```python
from build123d import *

# Parameters (mm, degrees)
SKETCH1_R           = 4.75
SKETCH1_R_2         = 1.5
BOSS_EXTRUDE1_DEPTH = 2
CHAMFER1_SIZE       = 1.5


with BuildPart() as part:
    # Sketch1 → Boss-Extrude1 (new body)
    with BuildSketch(Plane(origin=(0, 0, 0), x_dir=(1, 0, 0), z_dir=(0, 1, 0))):
        with BuildLine():
            Line((3.5, 17), (3.5, 9.5))
            ThreePointArc((3.5, 9.5), (5.257359313, 5.257359313), (9.5, 3.5))
            Line((9.5, 3.5), (17, 3.5))
            ThreePointArc((17, 3.5), (20.5, 0), (17, -3.5))
            Line((17, -3.5), (9.5, -3.5))
            ThreePointArc((9.5, -3.5), (5.257359313, -5.257359313), (3.5, -9.5))
            Line((3.5, -9.5), (3.5, -17))
            ThreePointArc((3.5, -17), (0, -20.5), (-3.5, -17))
            Line((-3.5, -17), (-3.5, -9.5))
            ThreePointArc((-3.5, -9.5), (-5.257359313, -5.257359313), (-9.5, -3.5))
            Line((-9.5, -3.5), (-17, -3.5))
            ThreePointArc((-17, -3.5), (-20.5, 0), (-17, 3.5))
            Line((-17, 3.5), (-9.5, 3.5))
            ThreePointArc((-9.5, 3.5), (-5.257359313, 5.257359313), (-3.5, 9.5))
            Line((-3.5, 9.5), (-3.5, 17))
            ThreePointArc((-3.5, 17), (0, 20.5), (3.5, 17))
        make_face()
        Circle(SKETCH1_R, mode=Mode.SUBTRACT)
        with Locations((0, 8)):
            Circle(SKETCH1_R_2, mode=Mode.SUBTRACT)
        with Locations((0, 17)):
            Circle(SKETCH1_R_2, mode=Mode.SUBTRACT)
        with Locations((17, 0)):
            Circle(SKETCH1_R_2, mode=Mode.SUBTRACT)
        with Locations((9.5, 0)):
            Circle(SKETCH1_R_2, mode=Mode.SUBTRACT)
        with Locations((0, -17)):
            Circle(SKETCH1_R_2, mode=Mode.SUBTRACT)
        with Locations((0, -8)):
            Circle(SKETCH1_R_2, mode=Mode.SUBTRACT)
        with Locations((-17, 0)):
            Circle(SKETCH1_R_2, mode=Mode.SUBTRACT)
        with Locations((-9.5, 0)):
            Circle(SKETCH1_R_2, mode=Mode.SUBTRACT)
    extrude(amount=BOSS_EXTRUDE1_DEPTH)

    # Chamfer1
    chamfer1_edges = [part.edges().sort_by_distance(p)[0] for p in [
        (-1.5, 2, -8),
        (8, 2, 0),
        (-1.5, 2, 8),
        (-11, 2, 0),
    ]]
    chamfer(chamfer1_edges, length=CHAMFER1_SIZE)


solid = part.part
```
The listing builds one solid part. Answer for the finished solid, in the listing's coordinates (mm). A direction names the side the tool comes from. Coordinates: 2 decimals unless noted, no trailing zeros. Loops run counter-clockwise (first coordinate to the right, second up) from the corner with the lowest first, then second, coordinate; pieces in that order, holes last. Notation, with made-up numbers: (30.5, 57.25) -> (81.5, 57.25) arc R25 cw to (81.5, 79.25) -> close; hole circle Ø1 at (20, -10.5). An arc over 180 degrees is marked (long way). Use one line per item in the form item = value. Start each with the question number.
Item 1: The part is cut by section B-B on x = -18. Determine the outline of the cut face in (y, z).
Item 2: The part is cut by section C-C on z = -8. Determine the outline of the cut face in (x, y).
Item 3: Flat-ended cylindrical pins translate along their axes: pin 1 Ø2.5 at (x, z) = (0, -17) entering from -Y; pin 2 Ø1 at (x, y) = (15, 1) entering from -Z; pin 3 Ø4 at (x, z) = (-17, 0) entering from +Y; pin 4 Ø0.6 at (y, z) = (1.5, -14) entering from -X. Find the tip coordinate at first contact, or state that the pin passes through.
Item 4: The mould has two halves that part along X. Classify faces 6 (the face through (-20.5, 1, 0.1)), 7 (the face through (0, 1, 6)), 8 (the face through (5, 0, -2)): released by +X, released by -X, zero draft, split by the parting line, or undercut.
Item 5: A tool of negligible diameter and unlimited length cuts with its end or side. For faces 1 (the face through (-11, 0.25, -0.07)), 2 (the face through (-13, 1, -3.5)), 3 (the face through (3.5, 1, -13)), 4 (the face through (3.5, 1, 13)), 5 (the face through (-13, 1, 3.5)), from which of +Z, -Z, +X, -X, +Y, -Y can it reach the whole face along a straight path? Write none if from no direction.
Item 6: The part is cut by section A-A on y = 0.85. Count the separate pieces of the cut face and the enclosed holes in it, then the cut area to 3 significant figures.
Item 7: Consider L1, parallel to Z at x = 0.5, y = 0.85; L2, parallel to Z at x = -17, y = 0.1; L3, parallel to X at y = 0.35, z = -8. Determine where each line is inside the solid, lowest interval first. Write a range as [from, to].
Item 8: The part is cut by section D-D on x = 16.5. Determine the outline of the cut face in (y, z).
Answer key:
q1.outline = (0, -3.35) -> (2, -3.35) -> (2, -1.12) -> (0, -1.12) -> close; (0, 1.12) -> (2, 1.12) -> (2, 3.35) -> (0, 3.35) -> close
q2.outline = (-3.69, 0) -> (-1.5, 0) -> (-1.5, 0.5) -> (-3, 2) -> (-3.69, 2) -> close; (1.5, 0) -> (3.69, 0) -> (3.69, 2) -> (3, 2) -> (1.5, 0.5) -> close
q3.pin_1 = through
q3.pin_2 = -3.5
q3.pin_3 = 2
q3.pin_4 = -3.5
q4.face_6 = released by -X
q4.face_7 = undercut
q4.face_8 = zero draft
q5.face_1 = +Y, -Y
q5.face_2 = -Z, -X, +Y, -Y
q5.face_3 = -Z, +X, +Y, -Y
q5.face_4 = +Z, +X, +Y, -Y
q5.face_5 = +Z, -X, +Y, -Y
q6.separate_pieces = 1
q6.enclosed_holes = 9
q6.area = 393 mm2
q7.L1 = [-20.46, -18.41], [-15.59, -9.78], [-6.22, -4.72], [4.72, 6.22], [9.78, 15.59], [18.41, 20.46]
q7.L2 = [-3.5, -1.5], [1.5, 3.5]
q7.L3 = [-3.69, -1.5], [1.5, 3.69]
q8.outline = (0, -3.5) -> (2, -3.5) -> (2, -1.41) -> (0, -1.41) -> close; (0, 1.41) -> (2, 1.41) -> (2, 3.5) -> (0, 3.5) -> close
